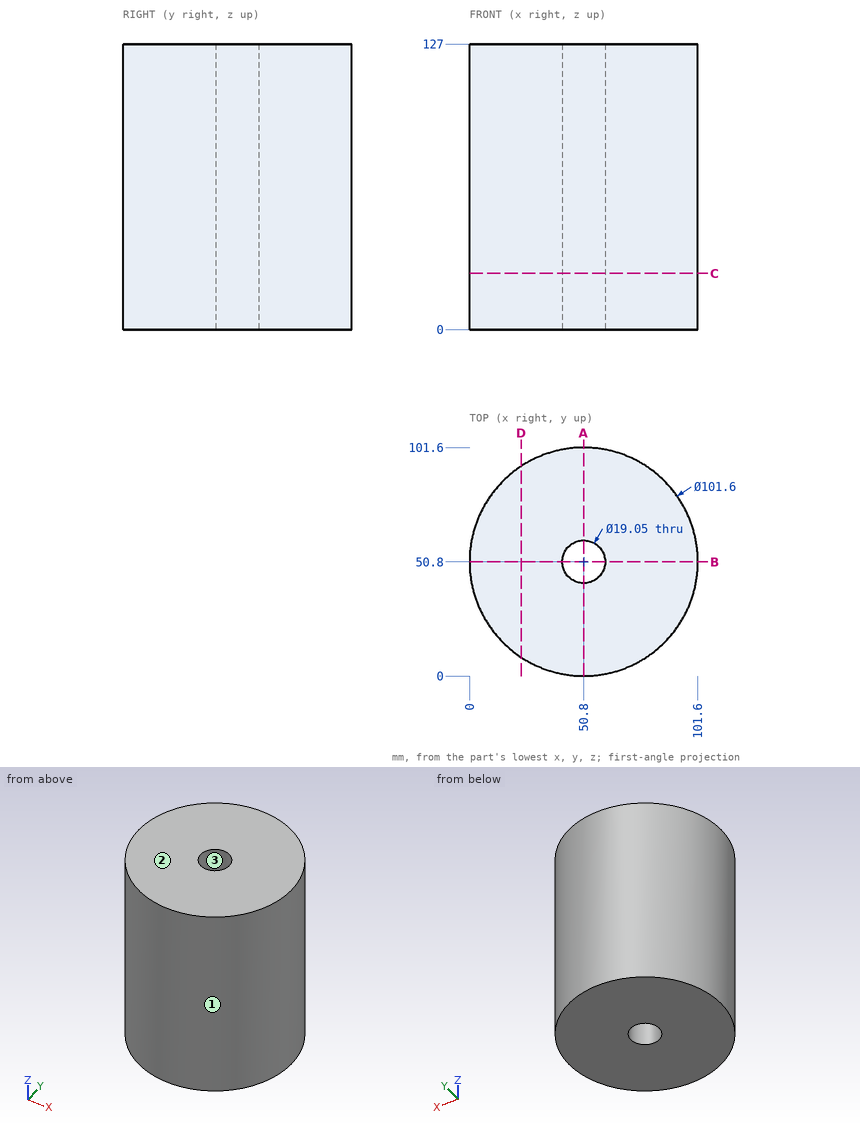
Check sheet for the drawn part. Datum: minimum x, y, z corner. Units: mm. Round coordinates to 2 decimals unless told otherwise and drop trailing zeros. Order: outer loops, then holes, each group sorted by start corner. A loop starts at its lowest first (then second) coordinate and runs counter-clockwise, first axis right, second up. Notation, with made-up numbers: M 31.5,73 L 41.5,73 A15 cw 41.5,98 Z; hole C -37,72.5 d8. An arc over 180 degrees is marked long. Write each question's results on one line, items separated by ' | '. Start each with the question number.
1. Cross-section at A-A on x = 50.8. Record the boundary of the cut face in (y, z) (3 decimals).
2. Material ranges on L1, parallel to X at y = 50, z = 53; L2, parallel to Y at x = 50.8, z = 46 (3 decimals); L3, parallel to Y at x = 90.5, z = 5, recorded low to high. Write a range as from..to.
3. Draft check along X on the marked faces 1, 2 and 3. Enter one of: pulls with the +X half, pulls with the -X half, needs draft (parallel to the pull), parting line crosses it, or undercut.
4. Cross-section at D-D on x = 23. Record the boundary of the cut face in (y, z), plus the area to 3 significant figures.
5. Cross-section at C-C on z = 25. Record the boundary of the cut face in (x, y) (3 decimals).
6. Go/stop test with flat-tipped pins: P1, Ø5, axis at y = 12, z = 21, coming from the +X side; P2, Ø1.5, axis at y = 32.5, z = 44, coming from the -X side; P3, Ø6, axis at x = 58, z = 42, coming from the -Y side; P4, Ø1, axis at x = 56, y = 25.5, coming from the -Z side. Record where each tip stops, or that it passes through.
Resolved:
1) outline: M 0,0 L 41.275,0 L 41.275,127 L 0,127 Z; M 60.325,0 L 101.6,0 L 101.6,127 L 60.325,127 Z
2) L1: 0.01..41.31, 60.29..101.59 | L2: 0..41.275, 60.325..101.6 | L3: 19.11..82.49
3) face 1: parting line crosses it | face 2: needs draft | face 3: undercut
4) outline: M 8.28,0 L 93.32,0 L 93.32,127 L 8.28,127 Z | area: 10,800 mm2
5) outline: C 50.8,50.8 d101.6; hole C 50.8,50.8 d19.05
6) P1: x = 86.34 | P2: x = 3.13 | P3: y = 0.17 | P4: z = 0
